Verification items for the finished model (mm, model axes). A direction names the side the tool comes from. Coordinates: 2 decimals unless noted, no trailing zeros. Write each loop counter-clockwise with the first axis right and the second up, starting at its lowest first coordinate (ties: lowest second). Pieces come first, ordered by that corner, then holes. Notation, with made-up numbers: (36, 65.25) -> (53, 65.25) arc R19 ccw to (53, 81.25) -> close; hole circle Ø11 at (55, 11). An arc over 180 degrees is marked (long way). Write item = value, one per line. Start each with the question number.
(1) Gauge pin test, flat ends, axial feed: pin 1 Ø6 at (x, z) = (3, 68.5) entering from -Y; pin 2 Ø3 at (y, z) = (-1.5, 74) entering from +X; pin 3 Ø12 at (x, z) = (-11.5, 2) entering from +Y; pin 4 Ø3 at (y, z) = (-1, 74.5) entering from -X. Record the tip position at first contact, or that the pin passes through.
(2) Section check A-A (z = 27). Record the cut outline in (x, y), plus the area to 3 significant figures.
(3) Section check B-B (x = 33). Record the cut outline in (y, z), plus the area to 3 significant figures.
(4) Material ranges on probe 1 along X at (y, z) = (-5.25, 53); probe 2 along Y at (x, z) = (38, 54); probe 3 along Y at (x, z) = (9.5, 64), recorded low to high. Write a range as [from, to].
(5) Mould release check, pull along Y, two halves, no side actions. Record for faces 3 (the face through (-3, -9, -58.026)), 4 (the face through (-3, 0, -1)), 5 (the face through (-2, -17, 60.851)), 6 (the face through (39.197, -9, 1)): released by +Y, released by -Y, zero draft, split by the parting line, or undercut.
(6) Set-up check for faces 1 (the face through (41.737, -9, -1)), 2 (the face through (-43.75, -9, 1)): record each of +Z, -Z, +X, -X, +Y, -Y from which the full face is reachable in a straight line by a thin tool's end or side.
(7) Section check C-C (y = -7.75). Record the cut outline in (x, z), plus the area to 3 significant figures.
```python
from build123d import *

# Parameters (mm, degrees)
F0_W     = 88.027496
F0_H     = 121.417232
F1_DEPTH = 19.05
F2_T     = -2.54
F3_W     = 32.993815
F3_H     = 30.100085
F4_DEPTH = 2.54


with BuildPart() as f1:
    # F0 (on Front) → F1 (new body)
    with BuildSketch(Plane.XZ):
        with Locations((-2.276575, 0.142578)):
            Rectangle(F0_W, F0_H)
    extrude(amount=F1_DEPTH)

    # F2
    f2_openings = [f1.faces().sort_by_distance(p)[0] for p in [
        (-2.276575, -9.525, 60.851194),
    ]]
    offset(amount=F2_T, openings=f2_openings)

    # F3 (on face) → F4 (join)
    with BuildSketch(Plane.XZ):
        with Locations((-1.319751, 75.901236)):
            Rectangle(F3_W, F3_H)
    extrude(amount=F4_DEPTH)


solid = f1.part
```
Response:
q1.pin_1 = -2.54
q1.pin_2 = 15.18
q1.pin_3 = 0
q1.pin_4 = -17.82
q2.outline = (-46.29, -19.05) -> (41.74, -19.05) -> (41.74, 0) -> (-46.29, 0) -> close; hole (-43.75, -16.51) -> (39.2, -16.51) -> (39.2, -2.54) -> (-43.75, -2.54) -> close
q2.area = 518 mm2
q3.outline = (-19.05, -60.57) -> (0, -60.57) -> (0, 60.85) -> (-2.54, 60.85) -> (-2.54, -58.03) -> (-16.51, -58.03) -> (-16.51, 60.85) -> (-19.05, 60.85) -> close
q3.area = 652 mm2
q4.probe_1 = [-46.29, -43.75], [39.2, 41.74]
q4.probe_2 = [-19.05, -16.51], [-2.54, 0]
q4.probe_3 = [-2.54, 0]
q5.face_3 = undercut
q5.face_4 = released by +Y
q5.face_5 = zero draft
q5.face_6 = undercut
q6.face_1 = +Z, -Z, +X, +Y, -Y
q6.face_2 = +Z
q7.outline = (-46.29, -60.57) -> (41.74, -60.57) -> (41.74, 60.85) -> (39.2, 60.85) -> (39.2, -58.03) -> (-43.75, -58.03) -> (-43.75, 60.85) -> (-46.29, 60.85) -> close
q7.area = 827 mm2
